from build123d import *

# Parameters (mm, degrees)
F1_DEPTH = 25.4


with BuildPart() as f1:
    # F0 (on Front) → F1 (new body, symmetric)
    with BuildSketch(Plane.XZ):
        Polygon((-28.572113, 33.450269), (0, 0), (0, 43.027113), align=None)
        Polygon((22.983828, 37.510396), (0, 0), (40.642365, 16.836993), align=None)
        Polygon((42.7769, -10.267569), (0, 0), (28.572113, -33.450269), align=None)
        Polygon((0, 0), (-22.983828, -37.510396), (3.45375, -43.856103), align=None)
        Polygon((-42.7769, 10.267569), (-40.642365, -16.836993), (0, 0), align=None)
        Polygon((-42.7769, 10.267569), (0, 0), (-28.572113, 33.450269), align=None)
        Polygon((0, 43.027113), (0, 0), (22.983828, 37.510396), align=None)
        Polygon((40.642365, 16.836993), (0, 0), (42.7769, -10.267569), align=None)
        Polygon((0, 0), (3.45375, -43.856103), (28.572113, -33.450269), align=None)
        Polygon((-40.642365, -16.836993), (-22.983828, -37.510396), (0, 0), align=None)
    extrude(amount=F1_DEPTH, both=True)


solid = f1.part
Source: CAD feature listing. Evaluate the final solid. Frame: model axes, mm. Coordinates: 2 decimals unless noted, no trailing zeros. Loops run counter-clockwise (first coordinate to the right, second up) from the corner with the lowest first, then second, coordinate; pieces in that order, holes last. Notation, with made-up numbers: (-25.75, 21.25) -> (23.25, 21.25) arc R21 cw to (23.25, 45.25) -> close; hole circle Ø6 at (32.25, -12). An arc over 180 degrees is marked (long way). Answer in a Markdown table with one row per item. Add a question column.
Q1. Contact query for flat-ended pins moving along their axis: pin 1 Ø1 at (y, z) = (16, 11.5) entering from -X; pin 2 Ø5 at (y, z) = (-19.5, 27) entering from +X; pin 3 Ø3 at (y, z) = (17.5, 8.5) entering from -X. Output: stop coordinate, or through.
Q2. Section A-A on y = -2.5. Return the cut outline in (x, z).
Q3. Section B-B on x = -20. Return the cut outline in (y, z), and give its area (3 significant figures).
Q4. Ray query, line 1 along Z through (x, y) = (-14, -1.5); line 2 along Z through (x, y) = (17.5, -11); line 3 along X through (y, z) = (-14.5, -0.5). Return the intervals inside material, ascending.
Q5. Section C-C on z = 31. Return the cut outline in (x, y), and give its area (3 significant figures).
Computed values:
| question | item | result |
|---|---|---|
| 1 | pin 1 | stops at x = -42.33 |
| 1 | pin 2 | stops at x = 34.1 |
| 1 | pin 3 | stops at x = -42.76 |
| 2 | outline | (-42.78, 10.27) -> (-40.64, -16.84) -> (-22.98, -37.51) -> (3.45, -43.86) -> (28.57, -33.45) -> (42.78, -10.27) -> (40.64, 16.84) -> (22.98, 37.51) -> (0, 43.03) -> (-28.57, 33.45) -> close |
| 3 | outline | (-25.4, -38.23) -> (25.4, -38.23) -> (25.4, 36.32) -> (-25.4, 36.32) -> close |
| 3 | area | 3,790 mm^2 |
| 4 | line 1 | z = -39.67 to 38.33 |
| 4 | line 2 | z = -38.04 to 38.83 |
| 4 | line 3 | x = -41.93 to 42.01 |
| 5 | outline | (-30.07, -25.4) -> (28.54, -25.4) -> (28.54, 25.4) -> (-30.07, 25.4) -> close |
| 5 | area | 2,980 mm^2 |
